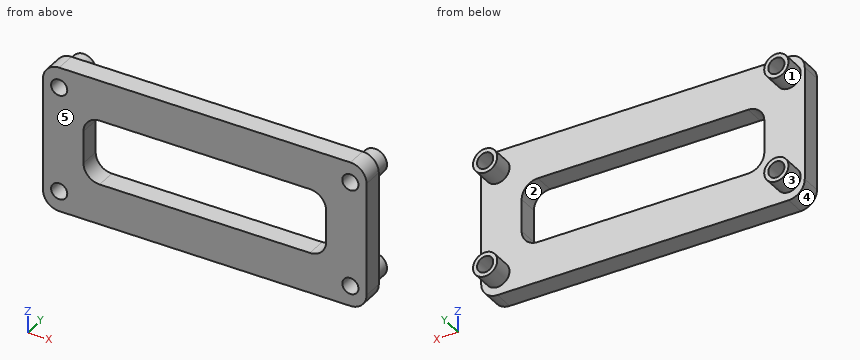
```python
from build123d import *

# Parameters (mm, degrees)
SKETCH1_W           = 50.8
SKETCH1_H           = 22.86
SKETCH1_R           = 1.27
SKETCH1_W_2         = 38.1
SKETCH1_H_2         = 10.16
BOSS_EXTRUDE1_DEPTH = 3.175
SKETCH2_R           = 1.905
SKETCH2_R_2         = 1.27
BOSS_EXTRUDE2_DEPTH = 3.175
FILLET1_R           = 2.54


with BuildPart() as part:
    # Sketch1 → Boss-Extrude1 (new body)
    with BuildSketch(Plane(origin=(0, 0, 0), x_dir=(1, 0, 0), z_dir=(0, 1, 0))):
        with Locations((25.4, 11.43)):
            Rectangle(SKETCH1_W, SKETCH1_H)
        with Locations((2.54, 19.685)):
            Circle(SKETCH1_R, mode=Mode.SUBTRACT)
        with Locations((48.26, 19.685)):
            Circle(SKETCH1_R, mode=Mode.SUBTRACT)
        with Locations((2.54, 3.175)):
            Circle(SKETCH1_R, mode=Mode.SUBTRACT)
        with Locations((48.26, 3.175)):
            Circle(SKETCH1_R, mode=Mode.SUBTRACT)
        with Locations((25.4, 11.43)):
            Rectangle(SKETCH1_W_2, SKETCH1_H_2, mode=Mode.SUBTRACT)
    extrude(amount=BOSS_EXTRUDE1_DEPTH)

    # Sketch2 → Boss-Extrude2 (add)
    with BuildSketch(Plane(origin=(0, 3.175, 0), x_dir=(1, 0, 0), z_dir=(0, 1, 0))):
        with Locations((2.54, 19.685)):
            Circle(SKETCH2_R)
        with Locations((2.54, 19.685)):
            Circle(SKETCH2_R_2, mode=Mode.SUBTRACT)
        with Locations((2.54, 3.175)):
            Circle(SKETCH2_R)
        with Locations((2.54, 3.175)):
            Circle(SKETCH2_R_2, mode=Mode.SUBTRACT)
        with Locations((48.26, 3.175)):
            Circle(SKETCH2_R)
        with Locations((48.26, 3.175)):
            Circle(SKETCH2_R_2, mode=Mode.SUBTRACT)
        with Locations((48.26, 19.685)):
            Circle(SKETCH2_R)
        with Locations((48.26, 19.685)):
            Circle(SKETCH2_R_2, mode=Mode.SUBTRACT)
    extrude(amount=BOSS_EXTRUDE2_DEPTH)

    # Fillet1
    fillet1_edges = [part.edges().sort_by_distance(p)[0] for p in [
        (6.35, 1.5875, -16.51),
        (6.35, 1.5875, -6.35),
        (44.45, 1.5875, -6.35),
        (44.45, 1.5875, -16.51),
        (0, 1.5875, -22.86),
        (50.8, 1.5875, -22.86),
        (50.8, 1.5875, 0),
        (0, 1.5875, 0),
    ]]
    fillet(fillet1_edges, radius=FILLET1_R)


solid = part.part
```
Geometry: final body of the model. Coordinates: model frame, mm. Face numbers are marked on the shaded views. A direction names the side the tool comes from. Coordinates: 2 decimals unless noted, no trailing zeros. Order: outer loops, then holes, each group sorted by start corner. A loop starts at its lowest first (then second) coordinate and runs counter-clockwise, first axis right, second up. Notation, with made-up numbers: (-30, 4) -> (29, 4) arc R12 ccw to (29, 22) -> close; hole circle Ø9 at (-13.75, -16.5). An arc over 180 degrees is marked (long way). Write each question's results on one line, items separated by ' | '. Start each with the question number.
1) Mould query, pull axis X, two halves, no side actions, for the marked faces 3, 4 and 5. Classes: released by +X, released by -X, zero draft, split by the parting line, or undercut.
2) First-contact query: pin 1 (4 mm diameter, centred on x = 2.54, z = -19.685, fed in from -Y); pin 2 (7 mm diameter, centred on x = 17.5, z = -16, fed in from +Y) (3 decimals); pin 3 (1.5 mm diameter, centred on x = 48.26, z = -3.175, fed in from -Y). Flat tips, straight axial feed; report the tip coordinate or a pass-through.
3) Material intervals for line 1 along Z through (x, y) = (2.54, 4.5) (3 decimals); line 2 along Z through (x, y) = (48.26, 2.25) (3 decimals); line 3 along Z through (x, y) = (21, 0.5), sorted ascending.
4) Cut plane A-A, the plane x = 40. Output: boundary loops of the cut face in (y, z) (3 decimals), and give its area (3 significant figures).
5) Cut plane D-D, the plane y = 1.25. Output: boundary loops of the cut face in (x, z) (3 decimals).
6) Cut plane C-C, the plane y = 5.75. Output: boundary loops of the cut face in (x, z) (3 decimals), and give its area (3 significant figures).
7) Set-up query: the marked faces 1 and 2. Return all of +Z, -Z, +X, -X, +Y, -Y with unobstructed straight access to the full face (end or side cutting, diameter ignored); none if empty.
8) Cut plane B-B, the plane z = -12. Output: boundary loops of the cut face in (x, y) (3 decimals), and give its area (3 significant figures).
Checks:
1) face 3: undercut | face 4: released by -X | face 5: zero draft
2) pin 1: y = 0 | pin 2: y = 3.175 | pin 3: through
3) line 1: -21.59 to -20.955, -18.415 to -17.78, -5.08 to -4.445, -1.905 to -1.27 | line 2: -22.86 to -20.955, -18.415 to -4.445, -1.905 to 0 | line 3: -22.86 to -16.51, -6.35 to 0
4) outline: (0, -22.86) -> (3.175, -22.86) -> (3.175, -16.51) -> (0, -16.51) -> close; (0, -6.35) -> (3.175, -6.35) -> (3.175, 0) -> (0, 0) -> close | area: 40.3 mm^2
5) outline: (0, -20.32) arc R2.54 ccw to (2.54, -22.86) -> (48.26, -22.86) arc R2.54 ccw to (50.8, -20.32) -> (50.8, -2.54) arc R2.54 ccw to (48.26, 0) -> (2.54, 0) arc R2.54 ccw to (0, -2.54) -> close; hole circle Ø2.54 at (2.54, -19.685); hole circle Ø2.54 at (2.54, -3.175); hole (6.35, -13.97) arc R2.54 ccw to (8.89, -16.51) -> (41.91, -16.51) arc R2.54 ccw to (44.45, -13.97) -> (44.45, -8.89) arc R2.54 ccw to (41.91, -6.35) -> (8.89, -6.35) arc R2.54 ccw to (6.35, -8.89) -> close; hole circle Ø2.54 at (48.26, -19.685); hole circle Ø2.54 at (48.26, -3.175)
6) outline: circle Ø3.81 at (2.54, -19.685); circle Ø3.81 at (2.54, -3.175); circle Ø3.81 at (48.26, -19.685); circle Ø3.81 at (48.26, -3.175); hole circle Ø2.54 at (2.54, -19.685); hole circle Ø2.54 at (2.54, -3.175); hole circle Ø2.54 at (48.26, -19.685); hole circle Ø2.54 at (48.26, -3.175) | area: 25.3 mm^2
7) face 1: +Y | face 2: +Y, -Y
8) outline: (0, 0) -> (6.35, 0) -> (6.35, 3.175) -> (0, 3.175) -> close; (44.45, 0) -> (50.8, 0) -> (50.8, 3.175) -> (44.45, 3.175) -> close | area: 40.3 mm^2
